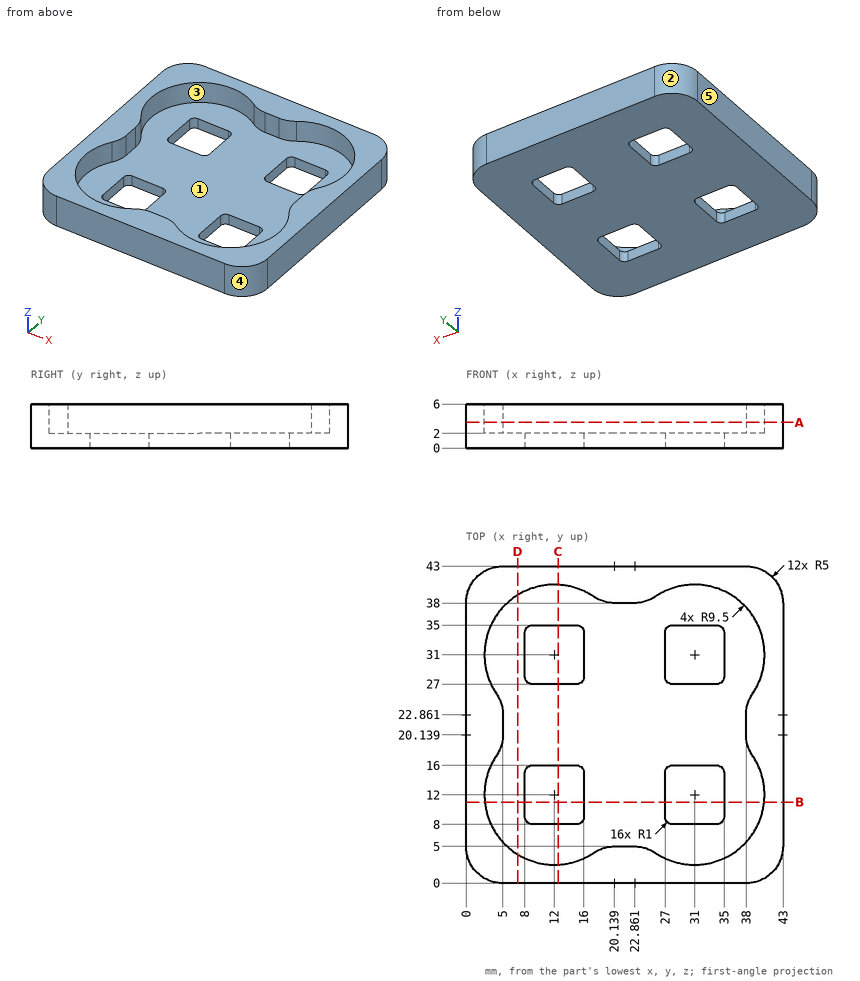
Geometry: see drawing. Coordinates: mm, zero at the bounding-box minimum. A direction names the side the tool comes from. Give positions to 0.01 mm unless a question says otherwise; leave off trailing zeros. Order: outer loops, then holes, each group sorted by start corner. A loop starts at its lowest first (then second) coordinate and runs counter-clockwise, first axis right, second up. Notation, with made-up numbers: M -2,-1 L 43,-1 A28 cw 43,35 Z; hole C -36,38.25 d9. An arc over 180 degrees is marked long. Answer as a JSON object with one key per item and string values.
1. Cut plane A-A, the plane z = 3.5. Output: boundary loops of the cut face in (x, y).
Result sheet:
{"outline": "M 0,5 A5 ccw 5,0 L 38,0 A5 ccw 43,5 L 43,38 A5 ccw 38,43 L 5,43 A5 ccw 0,38 Z; hole M 4.14,17.33 A9.5 ccw 17.33,4.14 A5 cw 20.14,5 L 22.86,5 A5 cw 25.67,4.14 A9.5 ccw 38.86,17.33 A5 cw 38,20.14 L 38,22.86 A5 cw 38.86,25.67 A9.5 ccw 25.67,38.86 A5 cw 22.86,38 L 20.14,38 A5 cw 17.33,38.86 A9.5 ccw 4.14,25.67 A5 cw 5,22.86 L 5,20.14 A5 cw Z"}
2. Reachability of the marked faces 1 and 2 from +Z, -Z, +X, -X, +Y, -Y: full face, straight path, thin tool, end or side. Return the list, or none.
Result sheet:
{"face 1": "+Z", "face 2": "+Z, -Z, -X, +Y"}
3. Pull-direction query (Y, two-part tool) for the marked faces 3, 4 and 5; classes: +Y half, -Y half, draft (parallel to the pull), parting line (faces both ways), or undercut.
Result sheet:
{"face 3": "undercut", "face 4": "-Y half", "face 5": "draft"}
4. First-contact query: P1, Ø11.5, axis at x = 23.5, y = 30, coming from the +Z side. Flat tip, straight axial feed; report the tip coordinate or a pass-through.
Result sheet:
{"P1": "z = 2"}
5. Cut plane D-D, the plane x = 7. Output: boundary loops of the cut face in (y, z).
Result sheet:
{"outline": "M 0,0 L 43,0 L 43,6 L 39.08,6 L 39.08,2 L 3.92,2 L 3.92,6 L 0,6 Z"}
6. Cut plane B-B, the plane y = 11. Output: boundary loops of the cut face in (x, z).
Result sheet:
{"outline": "M 0,0 L 8,0 L 8,2 L 2.55,2 L 2.55,6 L 0,6 Z; M 16,0 L 27,0 L 27,2 L 16,2 Z; M 35,0 L 43,0 L 43,6 L 40.45,6 L 40.45,2 L 35,2 Z"}
7. Ray query, line 1 (X direction, y = 14, z = 0.4); line 2 (X direction, y = 39, z = 5.3) (1 decimal). Return the intervals inside material, ascending. Write a range as [from, to].
Result sheet:
{"line 1": "[0, 8], [16, 27], [35, 43]", "line 2": "[0.1, 6.9], [17.1, 25.9], [36.1, 42.9]"}
8. Cut plane C-C, the plane x = 12.5. Output: boundary loops of the cut face in (y, z).
Result sheet:
{"outline": "M 0,0 L 8,0 L 8,2 L 2.51,2 L 2.51,6 L 0,6 Z; M 16,0 L 27,0 L 27,2 L 16,2 Z; M 35,0 L 43,0 L 43,6 L 40.49,6 L 40.49,2 L 35,2 Z"}
